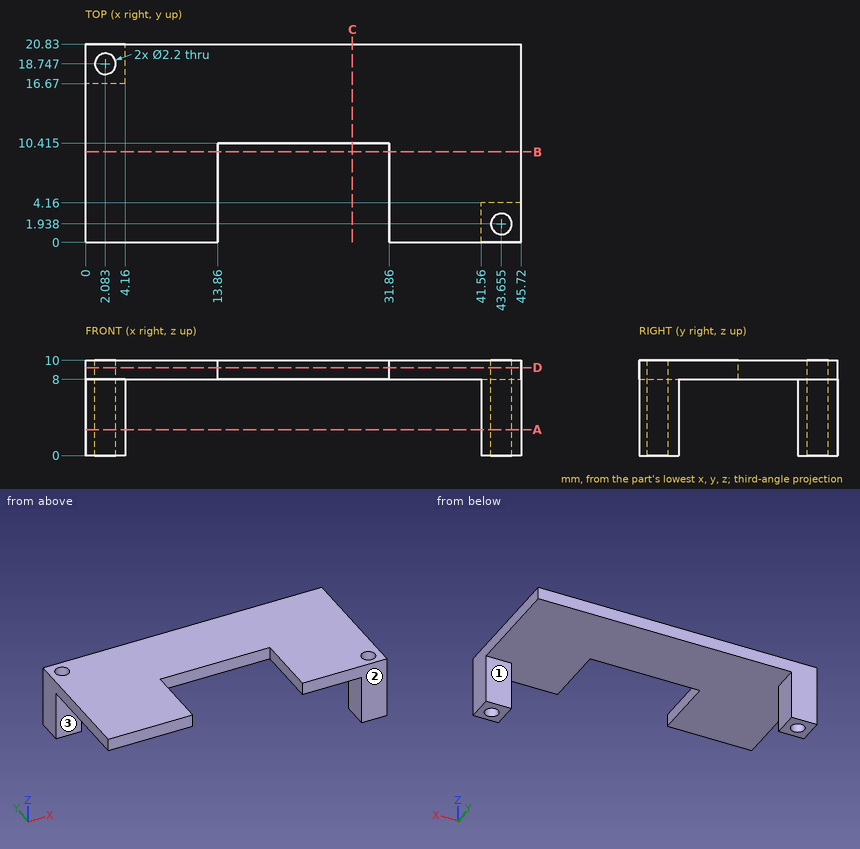
The figure shows three views and two pictorial views of one solid part (mm, origin at its lowest corner). Answer the questions. A direction names the side the tool comes from. Coordinates: 2 decimals unless noted, no trailing zeros. Loops run counter-clockwise (first coordinate to the right, second up) from the corner with the lowest first, then second, coordinate; pieces in that order, holes last. Notation, with made-up numbers: (23, 20.25) - (37, 20.25) arc R33 cw to (37, 48.25) - close; hole circle Ø8 at (16, 50.25). An arc over 180 degrees is marked (long way). Use a Markdown table: item, result. Add a question column.
1) Find the intervals of material crossed by line 1 (X direction, y = 6, z = 8.5); line 2 (Z direction, x = 41.5, y = 2.75); line 3 (X direction, y = 2.25, z = 2.5), in increasing order.
2) The part is cut by section C-C, the plane x = 28. Give the vertices of the cut face in (y, z) (1 decimal).
3) The part is cut by section B-B, the plane y = 9.5. Give the vertices of the cut face in (x, z).
4) The part is cut by section D-D, the plane z = 9.25. Give the vertices of the cut face in (x, y) (1 decimal), and give its area (3 significant figures).
5) The part is cut by section A-A, the plane z = 2.75. Give the vertices of the cut face in (x, y) (1 decimal).
6) For the marked faces 1, 2 and 3, determine the directions among +Z, -Z, +X, -X, +Y, -Y from which every point of the face is accessible in a straight line to the end or side of a thin tool.
7) Given pin 1 (2 mm diameter, centred on x = 43.5, z = 2.5, fed in from +Y); pin 2 (12 mm diameter, centred on x = 11, y = 8.5, fed in from -Z); pin 3 (1.5 mm diameter, centred on y = 5, z = 6.5, fed in from +X); pin 4 (2 mm diameter, centred on x = 1.5, z = 3.5, fed in from -Y), each flat-ended and moving along its own axis, determine where each tip first touches the part or whether it passes through.
Here are the results:
| question | item | result |
|---|---|---|
| 1 | line 1 | x = 0 to 13.86, 31.86 to 45.72 |
| 1 | line 2 | z = 8 to 10 |
| 1 | line 3 | x = 41.56 to 42.6, 44.71 to 45.72 |
| 2 | outline | (10.4, 8) - (20.8, 8) - (20.8, 10) - (10.4, 10) - close |
| 3 | outline | (0, 8) - (13.86, 8) - (13.86, 10) - (0, 10) - close; (31.86, 8) - (45.72, 8) - (45.72, 10) - (31.86, 10) - close |
| 4 | outline | (0, 0) - (13.9, 0) - (13.9, 10.4) - (31.9, 10.4) - (31.9, 0) - (45.7, 0) - (45.7, 20.8) - (0, 20.8) - close; hole circle Ø2.2 at (2.1, 18.7); hole circle Ø2.2 at (43.7, 1.9) |
| 4 | area | 757 mm^2 |
| 5 | outline | (0, 16.7) - (4.2, 16.7) - (4.2, 20.8) - (0, 20.8) - close; (41.6, 0) - (45.7, 0) - (45.7, 4.2) - (41.6, 4.2) - close; hole circle Ø2.2 at (2.1, 18.7); hole circle Ø2.2 at (43.7, 1.9) |
| 6 | face 1 | -Z, +X, -X, +Y |
| 6 | face 2 | +Z, -Z, +X, -X, -Y |
| 6 | face 3 | -Z, +X, -X, -Y |
| 7 | pin 1 | stops at y = 4.16 |
| 7 | pin 2 | stops at z = 8 |
| 7 | pin 3 | passes through |
| 7 | pin 4 | stops at y = 16.67 |
